Autodesk Fusion 360 part; units mm, degrees
sketch "Sketch1" plane through (0, 0, 0) normal (0, 0, 1) x (1, 0, 0)
  line L0 (0, 0) -> (80, 0)
  line L1 (80, 0) -> (80, 115)
  line L2 (80, 115) -> (0, 115)
  line L3 (0, 115) -> (0, 0)
  dimension "d1" = 80
  dimension "d2" = 115
sketch "Sketch2" plane through (0, 0, 0) normal (0, 0, 1) x (1, 0, 0)
extrude "Extrude1" add sketch "Sketch1" along normal blind 12
sketch "Sketch3" plane through (0, 0, 12) normal (0, 0, 1) x (-1, 0, 0)
  line L0 (0, -115) -> (0, 0)
  line L1 (0, 0) -> (-80, 0)
  line L2 (-80, 0) -> (-80, -115)
  line L3 (-80, -115) -> (0, -115)
  line L4 (0, -115) -> (-80, -115)
  line L5 (-80, -115) -> (-80, -57)
  line L6 (-80, -57) -> (0, -57)
  line L7 (0, -57) -> (0, -115)
  line L8 (-16, -57) -> (-64, -57)
  line L9 (-64, -57) -> (-64, -29)
  line L10 (-64, -29) -> (-16, -29)
  line L11 (-16, -29) -> (-16, -57)
  circle A0 centre (-40, -29) radius 24
  dimension "d5" = 58
  dimension "d6" = 48
  dimension "d7" = 28
extrude "Extrude2" add sketch "Sketch3" along normal blind 20 contours L0 L2 L3 L4 L5 L6 L7 L8 | L6 L8 L9 L11 A0 | L10 A0 | L10 A0
sketch "Sketch4" plane through (0, 0, 32) normal (0, 0, 1) x (-1, 0, 0)
  line L0 (-16, -57) -> (-16, -29)
  arc A0 (-16, -29) -> (-64, -29) centre (-40, -29) ccw
  line L1 (-64, -29) -> (-64, -57)
  line L2 (-64, -57) -> (-80, -57)
  line L3 (-80, -57) -> (-80, -115)
  line L4 (-80, -115) -> (0, -115)
  line L5 (0, -115) -> (0, -57)
  line L6 (0, -57) -> (-16, -57)
  line L7 (0, -115) -> (-80, -115)
  line L8 (-80, -115) -> (-80, -85)
  line L9 (-80, -85) -> (0, -85)
  line L10 (0, -85) -> (0, -115)
  line L11 (-40, -85) -> (-37.1656, -85)
  line L12 (-37.1656, -85) -> (-37.1656, -57)
  line L13 (-37.1656, -57) -> (-40, -57)
  line L14 (-40, -57) -> (-40, -85)
  line L15 (-37.1656, -57) -> (-45.1656, -57)
  line L16 (-45.1656, -57) -> (-45.1656, -85)
  line L17 (-45.1656, -85) -> (-37.1656, -85)
  line L18 (-37.1656, -85) -> (-37.1656, -57)
  dimension "d10" = 28
  dimension "d11" = 8
extrude "Extrude3" add sketch "Sketch4" along normal blind 24 contours L3 L4 L5 L7 L8 L9 L10 L11 L17 | L9 L11 L12 L13 L14 L15 L17 L18 | L9 L14 L15 L16 L17
sketch "Sketch5" plane through (37.1656, 0, 0) normal (-1, 0, 0) x (0, -1, 0)
  line L0 (-85, 32) -> (-57, 32)
  line L1 (-57, 32) -> (-57, 56)
  line L2 (-57, 56) -> (-85, 56)
  line L3 (-85, 56) -> (-85, 32)
  line L4 (-85, 56) -> (-57, 32)
  line L5 (-85, 56) -> (-57, 56)
  line L6 (-57, 32) -> (-57, 56)
extrude "Extrude4" cut sketch "Sketch5" against normal blind 8 contours L1 L2 L4 L5 L6
sketch "Sketch6" plane through (0, 0, 56) normal (0, 0, 1) x (-1, 0, 0)
  line L0 (-37.1656, -85) -> (-45.1656, -85)
  line L1 (-45.1656, -85) -> (-80, -85)
  line L2 (-80, -85) -> (-80, -115)
  line L3 (-80, -115) -> (0, -115)
  line L4 (0, -115) -> (0, -85)
  line L5 (0, -85) -> (-37.1656, -85)
  line L6 (0, -115) -> (-16, -115)
  line L7 (-16, -115) -> (-16, -105)
  line L8 (-16, -105) -> (-8, -105)
  line L9 (-8, -105) -> (-8, -95)
  line L10 (-80, -115) -> (-64, -115)
  line L11 (-64, -115) -> (-64, -105)
  line L12 (-64, -105) -> (-72, -105)
  line L13 (-72, -105) -> (-72, -95)
  line L14 (-72, -95) -> (-8, -95)
  line L15 (-16, -115) -> (-64, -115)
  dimension "d16" = 16
  dimension "d17" = 10
  dimension "d18" = 10
  dimension "d19" = 16
  dimension "d20" = 8
extrude "Extrude5" cut sketch "Sketch6" against normal blind 90 contours L3 L7 L8 L9 L11 L12 L13 L14 L15
sketch "Sketch7" plane through (0, 0, 32) normal (0, 0, 1) x (-1, 0, 0)
  line L0 (-80, -85) -> (-45.1656, -85)
  line L1 (-45.1656, -85) -> (-45.1656, -57)
  line L2 (-45.1656, -57) -> (-37.1656, -57)
  line L3 (-37.1656, -57) -> (-37.1656, -85)
  line L4 (-37.1656, -85) -> (0, -85)
  line L5 (0, -85) -> (0, -57)
  line L6 (0, -57) -> (-16, -57)
  line L7 (-16, -57) -> (-16, -29)
  arc A0 (-16, -29) -> (-64, -29) centre (-40, -29) ccw
  line L8 (-64, -29) -> (-64, -57)
  line L9 (-64, -57) -> (-80, -57)
  line L10 (-80, -57) -> (-80, -85)
  circle A1 centre (-40, -29) radius 17
  dimension "d23" = 34
extrude "Extrude6" cut sketch "Sketch7" against normal blind 5 contours A1
sketch "Sketch8" plane through (0, 0, 27) normal (0, 0, 1) x (-1, 0, 0)
  circle A0 centre (-40, -29) radius 17
  circle A1 centre (-40, -29) radius 12
  dimension "d26" = 24
extrude "Extrude7" cut sketch "Sketch8" against normal blind 49 contours A1
sketch "Sketch9" plane through (0, 0, 32) normal (0, 0, 1) x (-1, 0, 0)
  circle A0 centre (-40, -29) radius 17
  line L0 (-80, -85) -> (-45.1656, -85)
  line L1 (-45.1656, -85) -> (-45.1656, -57)
  line L2 (-45.1656, -57) -> (-37.1656, -57)
  line L3 (-37.1656, -57) -> (-37.1656, -85)
  line L4 (-37.1656, -85) -> (0, -85)
  line L5 (0, -85) -> (0, -57)
  line L6 (0, -57) -> (-16, -57)
  line L7 (-16, -57) -> (-16, -29)
  arc A1 (-16, -29) -> (-64, -29) centre (-40, -29) ccw
  line L8 (-64, -29) -> (-64, -57)
  line L9 (-64, -57) -> (-80, -57)
  line L10 (-80, -57) -> (-80, -85)
  circle A2 centre (-16, -71) radius 6
  circle A3 centre (-64, -71) radius 6
  dimension "d29" = 12
  dimension "d30" = 12
extrude "Extrude8" cut sketch "Sketch9" against normal blind 46 contours A2 | A3
Could you check a few things on this model? Use its own coordinates, in mm. A direction names the side the tool comes from. Coordinates: 2 decimals unless noted, no trailing zeros. Write each loop counter-clockwise with the first axis right and the second up, starting at its lowest first coordinate (ties: lowest second). Pieces come first, ordered by that corner, then holes. Notation, with made-up numbers: (76, 58.5) - (131, 58.5) arc R31 ccw to (131, 91.5) - close; hole circle Ø8 at (-30.5, 38.25). An arc over 180 degrees is marked (long way). Put each result on its own line as item: value. Start each with the question number.
Q1. I want a section at B-B on y = 71. Write out the boundary of the cut face in (x, z).
Q2. Thinking about a two-plate mould opening in Y: for faces 1 (the flat face through (72, 100, 28)), 2 (the flat face through (16, 110, 28)), 3 (the cylindrical face through (40.528, 5.006, 21.86)), which applies, pulls with the +Y half, pulls with the -Y half, needs draft (parallel to the pull), parting line crosses it, or undercut?
Q3. Which directions (+Z, -Z, +X, -X, +Y, -Y) give clear straight access to the entire face, cutting with the end or side of a thin tool? Please do faces 4 (the flat face through (16, 43, 22)), 5 (the flat face through (68, 105, 28)), 6 (the flat face through (63, 85, 44)).
Q4. I want a section at D-D on y = 38. Write out the boundary of the cut face in (x, z), plus the area to 3 significant figures.
Q5. I'm going to push flat-ended pins straight in: P1, Ø8, axis at y = 39.5, z = 28.5, coming from the -X side; P2, Ø17, axis at x = 36, y = 42, coming from the +Z side; P3, Ø2.5, axis at x = 68.5, z = 39.5, coming from the -Y side. Where does each tip first touch, or does it pass through?
Q6. I want a section at C-C on x = 40. Write out the boundary of the cut face in (y, z).
Q7. Please list where these lines run through material, in increasing order: L1, parallel to X at y = 71, z = 15; L2, parallel to Y at x = 70, z = 45; L3, parallel to X at y = 29, z = 29.85.
Q8. I want a section at A-A on z = 16. Write out the boundary of the cut face in (x, y).
Checks:
1. outline: (0, 0) - (10, 0) - (10, 32) - (0, 32) - close; (22, 0) - (58, 0) - (58, 32) - (45.17, 32) - (45.17, 44) - (37.17, 44) - (37.17, 32) - (22, 32) - close; (70, 0) - (80, 0) - (80, 32) - (70, 32) - close
2. face 1: undercut
2. face 2: needs draft
2. face 3: pulls with the -Y half
3. face 4: +Z, -X, -Y
3. face 5: +Z, -Z
3. face 6: +Z, +X, -Y
4. outline: (0, 0) - (32.06, 0) - (32.06, 27) - (25.58, 27) - (25.58, 32) - (16, 32) - (16, 12) - (0, 12) - close; (47.94, 0) - (80, 0) - (80, 12) - (64, 12) - (64, 32) - (54.42, 32) - (54.42, 27) - (47.94, 27) - close
4. area: 1,350 mm²
5. P1: x = 16
5. P2: z = 32
5. P3: y = 85
6. outline: (0, 0) - (17, 0) - (17, 27) - (12, 27) - (12, 32) - (5, 32) - (5, 12) - (0, 12) - close; (41, 0) - (95, 0) - (95, 56) - (85, 56) - (57, 32) - (46, 32) - (46, 27) - (41, 27) - close
7. L1: 0 to 10, 22 to 58, 70 to 80
7. L2: 85 to 95, 105 to 115
7. L3: 16 to 23, 57 to 64
8. outline: (0, 57) - (16, 57) - (16, 29) arc R24 ccw to (64, 29) - (64, 57) - (80, 57) - (80, 115) - (64, 115) - (64, 105) - (72, 105) - (72, 95) - (8, 95) - (8, 105) - (16, 105) - (16, 115) - (0, 115) - close; hole circle Ø12 at (16, 71); hole circle Ø24 at (40, 29); hole circle Ø12 at (64, 71)
